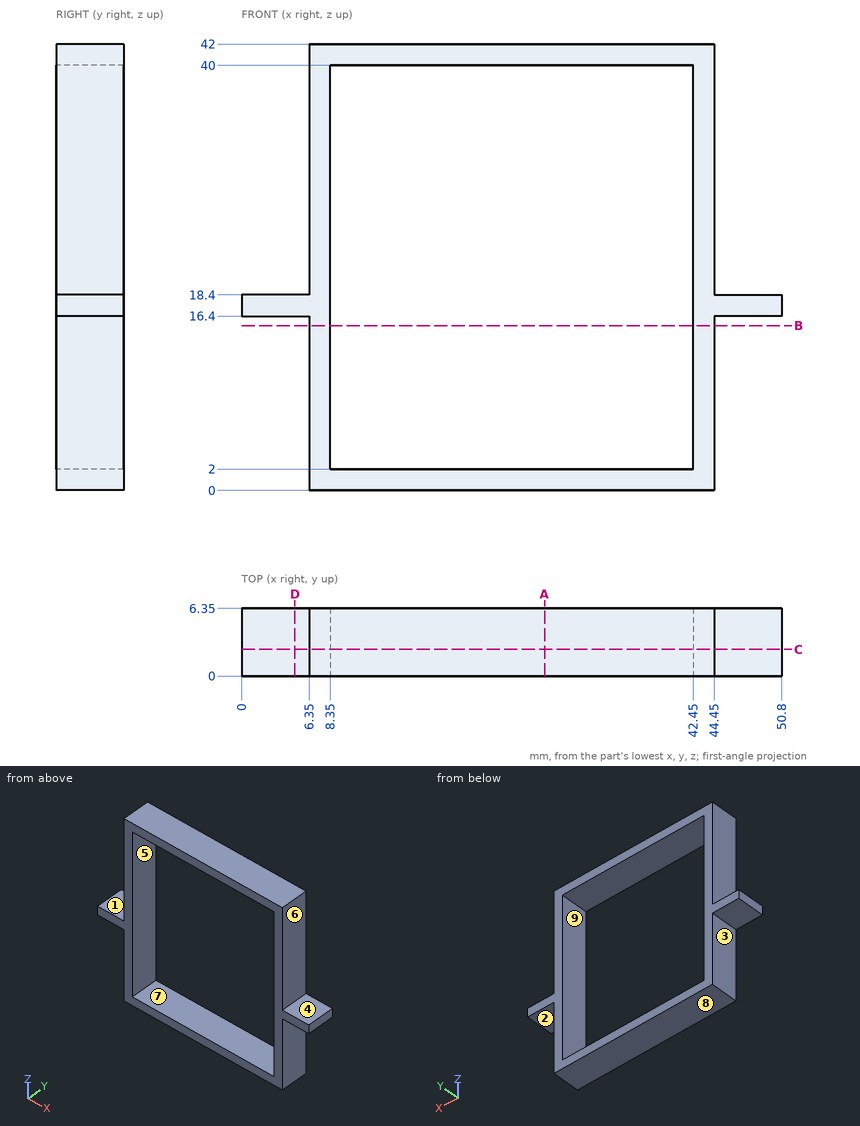
Input: dimensioned drawing with shaded views. Units: mm. Origin: part minimum x, y, z. A direction names the side the tool comes from. Round coordinates to 2 decimals unless told otherwise and drop trailing zeros. Loops run counter-clockwise (first coordinate to the right, second up) from the corner with the lowest first, then second, coordinate; pieces in that order, holes last. Notation, with made-up numbers: (73, 48.25) -> (95, 48.25) arc R17 cw to (95, 80.25) -> close; hole circle Ø3 at (26.5, -2). An arc over 180 degrees is marked (long way). One line per item, written item: value.
(1) Set-up query: the marked faces 1, 2, 3, 4 and 5. Return all of +Z, -Z, +X, -X, +Y, -Y with unobstructed straight access to the full face (end or side cutting, diameter ignored); none if empty.
Geometry check:
face 1: +Z, -X, +Y, -Y
face 2: -Z, +X, +Y, -Y
face 3: -Z, -X, +Y, -Y
face 4: +Z, +X, +Y, -Y
face 5: +Y, -Y
(2) Section A-A (x = 28.5). Return the cut outline in (y, z), plus the area to 3 significant figures.
Geometry check:
outline: (0, 0) -> (6.35, 0) -> (6.35, 2) -> (0, 2) -> close; (0, 40) -> (6.35, 40) -> (6.35, 42) -> (0, 42) -> close
area: 25.4 mm2
(3) Section C-C (y = 2.5). Return the cut outline in (x, z), plus the area to 3 significant figures.
Geometry check:
outline: (0, 16.4) -> (6.35, 16.4) -> (6.35, 0) -> (44.45, 0) -> (44.45, 16.4) -> (50.8, 16.4) -> (50.8, 18.4) -> (44.45, 18.4) -> (44.45, 42) -> (6.35, 42) -> (6.35, 18.4) -> (0, 18.4) -> close; hole (8.35, 2) -> (42.45, 2) -> (42.45, 40) -> (8.35, 40) -> close
area: 330 mm2
(4) Material intervals for line 1 (X direction, y = 3.25, z = 29); line 2 (Z direction, x = 11, y = 0.5); line 3 (Z direction, x = 5.5, y = 1), sorted ascending. Write a range as [from, to].
Geometry check:
line 1: [6.35, 8.35], [42.45, 44.45]
line 2: [0, 2], [40, 42]
line 3: [16.4, 18.4]
(5) Section B-B (z = 15.5). Return the cut outline in (x, y).
Geometry check:
outline: (6.35, 0) -> (8.35, 0) -> (8.35, 6.35) -> (6.35, 6.35) -> close; (42.45, 0) -> (44.45, 0) -> (44.45, 6.35) -> (42.45, 6.35) -> close
(6) Pin query (flat end, axial travel): pin 1 (3 mm diameter, centred on x = 35, y = 2.5, fed in from -Z); pin 2 (1.9 mm diameter, centred on y = 3.5, z = 29, fed in from +X); pin 3 (3 mm diameter, centred on x = 4.5, y = 4.5, fed in from -Z); pin 4 (3 mm diameter, centred on y = 2.5, z = 28.5, fed in from -X). Return the tip coordinate at first contact, or that it passes through.
Geometry check:
pin 1: z = 0
pin 2: x = 44.45
pin 3: z = 16.4
pin 4: x = 6.35
(7) Mould query, pull axis X, two halves, no side actions, for the marked faces 6, 7, 8 and 9. Classes: pulls with the +X half, pulls with the -X half, needs draft (parallel to the pull), parting line crosses it, or undercut.
Geometry check:
face 6: pulls with the +X half
face 7: undercut
face 8: needs draft
face 9: undercut
(8) Section D-D (x = 5). Return the cut outline in (y, z), plus the area to 3 significant figures.
Geometry check:
outline: (0, 16.4) -> (6.35, 16.4) -> (6.35, 18.4) -> (0, 18.4) -> close
area: 12.7 mm2
